Source: CAD feature listing. Evaluate the final solid. Frame: model axes, mm. A direction names the side the tool comes from. Give positions to 0.01 mm unless a question says otherwise; leave off trailing zeros. Order: outer loops, then holes, each group sorted by start corner. A loop starts at its lowest first (then second) coordinate and runs counter-clockwise, first axis right, second up. Notation, with made-up numbers: M 74.5,2 L 128.5,2 A23 cw 128.5,25 Z; hole C -28.5,-22 d9. An arc over 180 degrees is marked long. Answer in a Markdown table with one row per item. Add a question column.
(1) Set-up query: faces 4 (the face through (-70, 27, 38)), 5 (the face through (-65, 23, 38)), 6 (the face through (-4, 13, -40)), 7 (the face through (-65, 31.75, 29)), 8 (the face through (-40, 16, 12)). Return all of +Z, -Z, +X, -X, +Y, -Y with unobstructed straight access to the full face (end or side cutting, diameter ignored); none if empty.
(2) Section query A-A, the plane z = 35. Return loops of the section in (x, y) (3 decimals), plus the area to 3 significant figures.
(3) Material intervals for line 1 along Y through (x, z) = (-65.25, 35) (3 decimals); line 2 along Z through (x, y) = (-41.5, 29); line 3 along X through (y, z) = (29, 57), sorted ascending.
(4) Section query B-B, the plane y = 10. Return loops of the section in (x, z), plus the area to 3 significant figures.
(5) Section query C-C, the plane x = 0. Return loops of the section in (y, z), plus the area to 3 significant figures.
(6) Pin query (flat end, axial travel): P1, Ø4, axis at y = 27.375, z = 55, coming from the +X side; P2, Ø4.5, axis at x = -46.5, y = 26.5, coming from the +Z side; P3, Ø12, axis at y = 16, z = -31, coming from the -X side. Return the tip coordinate at first contact, or that it passes through.
(7) Mould query, pull axis Z, two halves, no side actions, for faces 1 (the face through (-52, 27, 25)), 2 (the face through (-64, 27, 45)), 3 (the face through (-66.96, 28.96, 35.21)). Classes: pulls with the +Z half, pulls with the -Z half, needs draft (parallel to the pull), parting line crosses it, or undercut.
(8) Section query D-D, the plane z = -14. Return loops of the section in (x, y), plus the area to 3 significant figures.
from build123d import *

# Parameters (mm, degrees)
EXTRUDE_1_DEPTH          = 13
SKETCH_2_W               = 30
SKETCH_2_H               = 13
EXTRUDE_2_DEPTH          = 5
EXTRUDE_3_DEPTH          = 30
SKETCH_4_W               = 30
SKETCH_4_H               = 8.75
EXTRUDE_4_DEPTH          = 10
CUT_EXTRUDE_3_DEPTH      = 86.302769592
CUT_EXTRUDE_3_DEPTH_BACK = 86.302769592
SKETCH_9_W               = 40
SKETCH_9_H               = 8.75
EXTRUDE_5_DEPTH          = 6
SKETCH_10_R              = 1.6
CUT_EXTRUDE_4_DEPTH      = 131.820726569
PATTERN_LINEAR_1_COUNT   = 2
PATTERN_LINEAR_1_PITCH   = 20
CHAMFER_3_SIZE           = 30
CHAMFER_3_SIZE_2         = 6.247089083
FILLET_1_R               = 20


with BuildPart() as part:
    # 草圖1 → 填料-伸長1 (new body)
    with BuildSketch(Plane(origin=(0, 0, 0), x_dir=(1, 0, 0), z_dir=(0, 1, 0))):
        with BuildLine():
            Line((-45, 0), (-40, 0))
            ThreePointArc((-40, 0), (0, 40), (40, 0))
            Line((40, 0), (45, 0))
            ThreePointArc((45, 0), (0, 45), (-45, 0))
        make_face()
    extrude(amount=EXTRUDE_1_DEPTH)

    # 草圖2 → 填料-伸長2 (add)
    with BuildSketch(Plane.XY):
        with Locations((-55, 6.5)):
            Rectangle(SKETCH_2_W, SKETCH_2_H)
    extrude(amount=EXTRUDE_2_DEPTH)

    # 草圖3 → 填料-伸長3 (add)
    with BuildSketch(Plane(origin=(-40, 0, 0), x_dir=(0, 0, -1), z_dir=(1, 0, 0))):
        Polygon((-5, 0), (-5, 13), (-15, 31.75), (-15, 23), align=None)
    extrude(amount=-EXTRUDE_3_DEPTH)

    # 草圖4 → 填料-伸長4 (add)
    with BuildSketch(Plane.XY.offset(15)):
        with Locations((-55, 27.375)):
            Rectangle(SKETCH_4_W, SKETCH_4_H)
    extrude(amount=EXTRUDE_4_DEPTH)

    # 草圖8 → 除料-伸長3 (cut, two sides: drawn at the far end of the back side and taken through both)
    with BuildSketch(Plane(origin=(0, 13, 0), x_dir=(1, 0, 0), z_dir=(0, 1, 0)).offset(-CUT_EXTRUDE_3_DEPTH_BACK)):
        Polygon((-45, 0), (-70, -15), (-70, 0), align=None)
    extrude(amount=CUT_EXTRUDE_3_DEPTH + CUT_EXTRUDE_3_DEPTH_BACK, mode=Mode.SUBTRACT)

    # 草圖9 → 填料-伸長5 (add)
    with BuildSketch(Plane.ZY.offset(70)):
        with Locations((45, 27.375)):
            Rectangle(SKETCH_9_W, SKETCH_9_H)
    extrude(amount=-EXTRUDE_5_DEPTH)

    # 草圖10 → 除料-伸長4 (cut, through all)
    with BuildSketch(Plane(origin=(-64, 0, 0), x_dir=(0, 0, -1), z_dir=(1, 0, 0))):
        with Locations((-35, 27.375)):
            Circle(SKETCH_10_R)
    cut_extrude_4 = extrude(amount=-CUT_EXTRUDE_4_DEPTH, mode=Mode.SUBTRACT)

    # 直線複製排列1: 除料-伸長4 ×2
    with Locations(*[(0, 0, i * PATTERN_LINEAR_1_PITCH) for i in range(1, PATTERN_LINEAR_1_COUNT)]):
        add(cut_extrude_4, mode=Mode.SUBTRACT)

    # 導角3
    # the kernel refuses this chamfer: 30, 6.247089083 mm, written as the material it adds along each edge
    with BuildSketch(Plane(origin=(-40, 23, 15), x_dir=(0, -0.9143850797176141, -0.4048455581944953), z_dir=(-1, 0, 0))) as chamfer_3_piece_1_section:
        Polygon((CHAMFER_3_SIZE * 0.999977671636, CHAMFER_3_SIZE * 0.0066825316561), (-CHAMFER_3_SIZE_2 * 0.404845558197, CHAMFER_3_SIZE_2 * 0.914385079723), (0, 0), align=None)
    chamfer_3_piece_1 = extrude(amount=30, mode=Mode.PRIVATE)
    chamfer_3_piece_1 = split(chamfer_3_piece_1, bisect_by=Plane(origin=(-53.38759528, 0, 13.91258777), z_dir=(0, 1, 0)), keep=Keep.TOP, mode=Mode.PRIVATE)
    chamfer_3_piece_1 = split(chamfer_3_piece_1, bisect_by=Plane(origin=(-57.305255839, 15.236001875, 7.383153504), z_dir=(0.5144957554275266, 0, 0.8574929257125442)), keep=Keep.TOP, mode=Mode.PRIVATE)
    add(chamfer_3_piece_1)

    # 圓角1
    fillet_1_edges = [part.edges().sort_by_distance(p)[0] for p in [
        (-45, 6.5, 0),
    ]]
    fillet(fillet_1_edges, radius=FILLET_1_R)


solid = part.part
Values follow:
| question | item | result |
|---|---|---|
| 1 | face 4 | +Z, -Z, -X, +Y, -Y |
| 1 | face 5 | +Z, +X, -X, -Y |
| 1 | face 6 | -Z, +X, -X, +Y |
| 1 | face 7 | +Z, -Z, +X, -X, +Y |
| 1 | face 8 | +Z, +X, +Y, -Y |
| 2 | outline | M -70,23 L -64,23 L -64,25.775 L -70,25.775 Z; M -70,28.975 L -64,28.975 L -64,31.75 L -70,31.75 Z |
| 2 | area | 33.3 mm² |
| 3 | line 1 | y = 23 to 25.775, 28.975 to 31.75 |
| 3 | line 2 | z = 13.53 to 25 |
| 3 | line 3 | x = -70 to -64 |
| 4 | outline | M -66.07,12.64 L -53.59,5.16 A20 cw -44.23,-8.3 A45 ccw 45,0 L 40,0 A40 cw -40,0 L -40,12.64 Z |
| 4 | area | 877 mm² |
| 5 | outline | M 0,-45 L 13,-45 L 13,-40 L 0,-40 Z |
| 5 | area | 65.0 mm² |
| 6 | P1 | stops at x = -64 |
| 6 | P2 | stops at z = 25 |
| 6 | P3 | stops at x = -36.87 |
| 7 | face 1 | pulls with the +Z half |
| 7 | face 2 | needs draft |
| 7 | face 3 | undercut |
| 8 | outline | M -42.77,0 L -37.47,0 L -37.47,13 L -42.77,13 Z; M 37.47,0 L 42.77,0 L 42.77,13 L 37.47,13 Z |
| 8 | area | 138 mm² |
